Geometry: final body of the model. Coordinates: model frame, mm. Give positions to 0.01 mm unless a question says otherwise; leave off trailing zeros. Order: outer loops, then holes, each group sorted by start corner. A loop starts at its lowest first (then second) coordinate and runs counter-clockwise, first axis right, second up. Notation, with made-up numbers: (2, -40) - (50, -40) arc R30 cw to (50, -3) - close; hole circle Ø11 at (45, 54). An arc over 180 degrees is marked (long way). Use one line per item in the form item = value.
from build123d import *

# Parameters (mm, degrees)
MAIN_PROFILE_SKETCH_R = 1.7
MAIN_EXTRUSION_DEPTH  = 3


with BuildPart() as part:
    # Main Profile Sketch → Main Extrusion (new body)
    with BuildSketch(Plane.XY.offset(44.5)):
        with BuildLine():
            Line((-130, 41.5), (-90, 41.5))
            Line((-90, 41.5), (-90, 31.5))
            Line((-90, 31.5), (-99.834359217, 31.5))
            ThreePointArc((-99.834359217, 31.5), (-102, 38.2), (-104.165640783, 31.5))
            Line((-104.165640783, 31.5), (-130, 31.5))
            Line((-130, 31.5), (-130, 41.5))
        make_face()
        with Locations((-125, 36.5)):
            Circle(MAIN_PROFILE_SKETCH_R, mode=Mode.SUBTRACT)
        with Locations((-95, 36.5)):
            Circle(MAIN_PROFILE_SKETCH_R, mode=Mode.SUBTRACT)
    extrude(amount=-MAIN_EXTRUSION_DEPTH)


solid = part.part
(1) Cut plane A-A on x = -125. Output: boundary loops of the cut face in (y, z), plus the area to 3 significant figures.
Computed values:
outline = (31.5, 41.5) - (34.8, 41.5) - (34.8, 44.5) - (31.5, 44.5) - close; (38.2, 41.5) - (41.5, 41.5) - (41.5, 44.5) - (38.2, 44.5) - close
area = 19.8 mm²
(2) Cut plane C-C on y = 36. Output: boundary loops of the cut face in (x, z).
Computed values:
outline = (-130, 41.5) - (-126.62, 41.5) - (-126.62, 44.5) - (-130, 44.5) - close; (-123.38, 41.5) - (-105.38, 41.5) - (-105.38, 44.5) - (-123.38, 44.5) - close; (-98.62, 41.5) - (-96.62, 41.5) - (-96.62, 44.5) - (-98.62, 44.5) - close; (-93.38, 41.5) - (-90, 41.5) - (-90, 44.5) - (-93.38, 44.5) - close
(3) Cut plane B-B on z = 43.4. Output: boundary loops of the cut face in (x, y).
Computed values:
outline = (-130, 31.5) - (-104.17, 31.5) arc R3.7 cw (long way) to (-99.83, 31.5) - (-90, 31.5) - (-90, 41.5) - (-130, 41.5) - close; hole circle Ø3.4 at (-125, 36.5); hole circle Ø3.4 at (-95, 36.5)
(4) Pull-direction query (Y, two-part tool) for faces 1 (the face through (-110, 41.5, 43)), 2 (the face through (-130, 36, 43)), 3 (the face through (-95, 31.5, 43)), 4 (the face through (-101.9, 38.2, 43)); classes: released by +Y, released by -Y, zero draft, split by the parting line, or undercut.
Computed values:
face_1 = released by +Y
face_2 = zero draft
face_3 = released by -Y
face_4 = undercut
(5) Ray query, line 1 along X through (y, z) = (37, 44.15); line 2 along X through (y, z) = (37.25, 42.6); line 3 along Y through (x, z) = (-95, 42.8). Return the intervals inside material, ascending.
Computed values:
line_1 = -130 to -126.62, -123.38 to -104.73, -99.27 to -96.62, -93.38 to -90
line_2 = -130 to -126.53, -123.47 to -104.48, -99.52 to -96.53, -93.47 to -90
line_3 = 31.5 to 34.8, 38.2 to 41.5
(6) Cut plane D-D on y = 33.25. Output: boundary loops of the cut face in (x, z), plus the area to 3 significant figures.
Computed values:
outline = (-130, 41.5) - (-105.48, 41.5) - (-105.48, 44.5) - (-130, 44.5) - close; (-98.52, 41.5) - (-90, 41.5) - (-90, 44.5) - (-98.52, 44.5) - close
area = 99.1 mm²
